Verification items for this drawing (mm, ordinates from the low corner). A direction names the side the tool comes from. Round coordinates to 2 decimals unless told otherwise and drop trailing zeros. Order: outer loops, then holes, each group sorted by start corner. A loop starts at its lowest first (then second) coordinate and runs counter-clockwise, first axis right, second up.
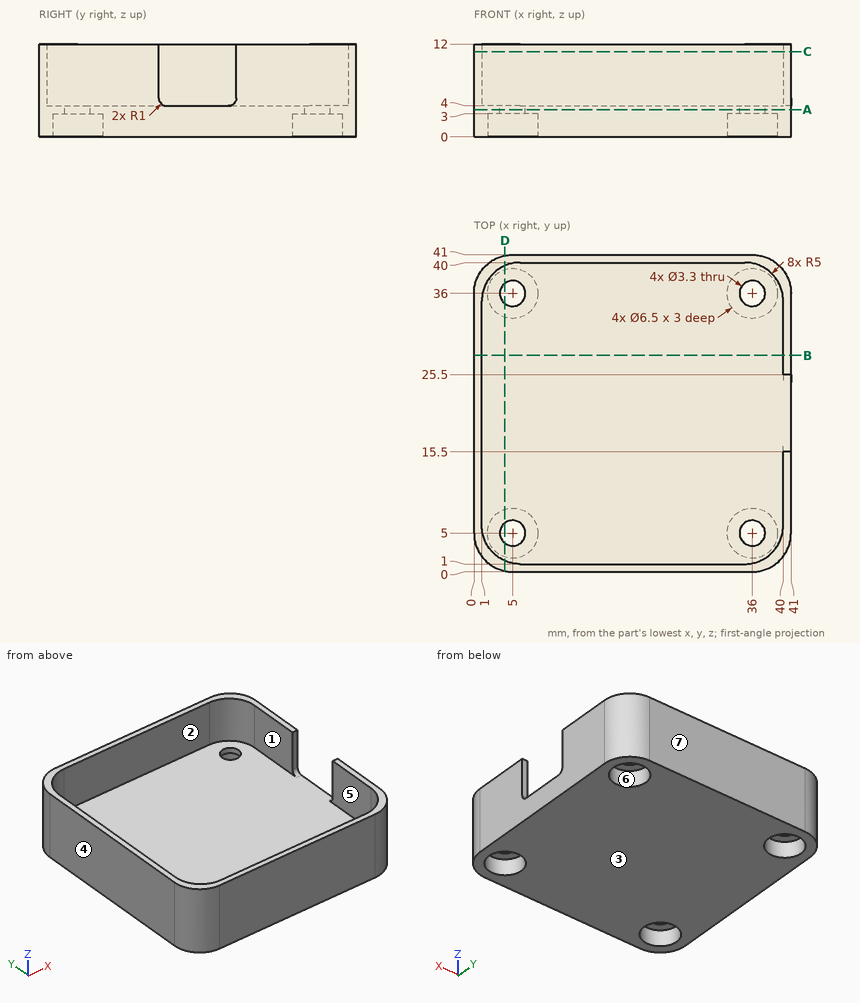
Item 1: Scan lines: line 1 along Y through (x, z) = (36, 3.4); line 2 along Y through (x, z) = (5, 2). Record each from-to range of solid material in increasing order.
Answer:
line 1: y = 0 to 3.35, 6.65 to 34.35, 37.65 to 41
line 2: y = 0 to 1.75, 8.25 to 32.75, 39.25 to 41
Item 2: Sectioned sample at C-C (z = 11). Record the cut outline in (x, y), and give its area (3 significant figures).
Answer:
outline: (0, 5) arc R5 ccw to (5, 0) - (36, 0) arc R5 ccw to (41, 5) - (41, 15.5) - (40, 15.5) - (40, 6) arc R5 cw to (35, 1) - (6, 1) arc R5 cw to (1, 6) - (1, 35) arc R5 cw to (6, 40) - (35, 40) arc R5 cw to (40, 35) - (40, 25.5) - (41, 25.5) - (41, 36) arc R5 ccw to (36, 41) - (5, 41) arc R5 ccw to (0, 36) - close
area: 150 mm2
Item 3: Access from +Z, -Z, +X, -X, +Y, -Y to the whole of each face (thin tool, end or side, straight path). Record for the marked faces 5, 6 and 7.
Answer:
face 5: +Z
face 6: -Z
face 7: +Z, -Z, +X, -X, +Y
Item 4: Go/stop test with flat-tipped pins: P1, Ø3, axis at x = 5, y = 36, coming from the -Z side; P2, Ø1, axis at x = 23.5, y = 25, coming from the +Z side; P3, Ø3, axis at x = 35.5, y = 4.5, coming from the -Z side; P4, Ø1.1, axis at x = 40.5, z = 8.5, coming from the -Y side. Record where each tip stops, or that it passes through.
Answer:
P1: passes through
P2: stops at z = 4
P3: stops at z = 3
P4: stops at y = 1.93
Item 5: Sectioned sample at A-A (z = 3.5). Record the cut outline in (x, y), and give its area (3 significant figures).
Answer:
outline: (0, 5) arc R5 ccw to (5, 0) - (36, 0) arc R5 ccw to (41, 5) - (41, 36) arc R5 ccw to (36, 41) - (5, 41) arc R5 ccw to (0, 36) - close; hole circle Ø3.3 at (5, 5); hole circle Ø3.3 at (5, 36); hole circle Ø3.3 at (36, 5); hole circle Ø3.3 at (36, 36)
area: 1,630 mm2
Item 6: Sectioned sample at D-D (x = 4). Record the cut outline in (y, z), and give its area (3 significant figures).
Answer:
outline: (0.1, 0) - (1.91, 0) - (1.91, 3) - (3.69, 3) - (3.69, 4) - (1.42, 4) - (1.42, 12) - (0.1, 12) - close; (6.31, 3) - (8.09, 3) - (8.09, 0) - (32.91, 0) - (32.91, 3) - (34.69, 3) - (34.69, 4) - (6.31, 4) - close; (37.31, 3) - (39.09, 3) - (39.09, 0) - (40.9, 0) - (40.9, 12) - (39.58, 12) - (39.58, 4) - (37.31, 4) - close
area: 142 mm2
Item 7: Release check for a two-part mould opening along X. For the marked faces 1, 2, 3 and 4 record: released by +X, released by -X, zero draft, split by the parting line, or undercut.
Answer:
face 1: undercut
face 2: undercut
face 3: zero draft
face 4: released by -X
Item 8: Sectioned sample at B-B (y = 28). Record the cut outline in (x, z).
Answer:
outline: (0, 0) - (41, 0) - (41, 12) - (40, 12) - (40, 4) - (1, 4) - (1, 12) - (0, 12) - close
